from build123d import *

# Parameters (mm, degrees)
SALIENTE_EXTRUIR1_DEPTH = 1.25
SALIENTE_EXTRUIR2_DEPTH = 3.25
SALIENTE_EXTRUIR3_DEPTH = 5
SALIENTE_EXTRUIR4_DEPTH = 225.499987602
SALIENTE_EXTRUIR6_REACH = 368.413
CROQUIS6_W              = 4.5
CROQUIS6_H              = 225.499987602
CHAFL_N1_SIZE           = 0.6
CHAFL_N1_SIZE_2         = 0.279784595
REDONDEO1_R             = 0.5
CORTAR_EXTRUIR1_REACH   = 369.581
CROQUIS8_R              = 1.7
CORTAR_EXTRUIR2_DEPTH   = 409.723751009


with BuildPart() as part:
    # Croquis1 → Saliente-Extruir1 (new body)
    with BuildSketch(Plane.XY):
        Polygon((287.750005722, 59.751000255), (272.747904062, 59.751000255), (267.749905586, 64.749002457), (64.157357861, 64.749002457), (64.553998411, 290.248990059), (76.149903238, 290.248990059), (76.149903238, 77.348701656), (276.148021221, 77.348701656), (276.148021221, 290.248990059), (287.750005722, 290.248990059), align=None)
    extrude(amount=SALIENTE_EXTRUIR1_DEPTH)

    # Croquis2 → Saliente-Extruir2 (add)
    with BuildSketch(Plane.XY.offset(1.25)):
        Polygon((286.75003751, 290.248990059), (287.750005722, 290.248990059), (287.750005722, 59.751000255), (272.747904062, 59.751000255), (267.749905586, 64.749002457), (64.157357861, 64.749002457), (64.553998411, 290.248990059), (65.547994841, 290.248990059), (65.547994841, 66.199905073), (286.75003751, 66.199905073), align=None)
    extrude(amount=SALIENTE_EXTRUIR2_DEPTH)

    # Croquis3 → Saliente-Extruir3 (add)
    with BuildSketch(Plane.XZ.offset(-64.749002457)):
        with BuildLine():
            Line((64.515409591, 0), (66.982480076, 0))
            ThreePointArc((66.982480076, 0), (65.748944833, 2.619014625), (64.515409591, 0))
        make_face()
    extrude(amount=SALIENTE_EXTRUIR3_DEPTH)

    # Saliente-Extruir6: up to this face of the body (flat: up to its plane)
    saliente_extruir6_end = Plane(part.part.faces().sort_by_distance((64.355678136, 177.498996258, 2.25))[0])
    # Croquis6 → Saliente-Extruir6 (add, up to the picked face)
    with BuildSketch(Plane(origin=(64.157357861, 0, 0), x_dir=(0, 0, -1), z_dir=(1, 0, 0)), mode=Mode.PRIVATE) as saliente_extruir6_sk1:
        with Locations((-2.25, 177.498996258)):
            Rectangle(CROQUIS6_W, CROQUIS6_H)
    saliente_extruir6_tool1 = split(extrude(saliente_extruir6_sk1.sketch, amount=SALIENTE_EXTRUIR6_REACH, mode=Mode.PRIVATE), bisect_by=saliente_extruir6_end, keep=Keep.BOTH, mode=Mode.PRIVATE)


with BuildPart() as body_2:
    # Croquis3<3> → Saliente-Extruir4 (new body)
    with BuildSketch(Plane.XZ.offset(-64.749002457)):
        with BuildLine():
            Line((64.157357861, 3.992626763), (64.157357861, 0))
            ThreePointArc((64.157357861, 0), (62.24843494, 1.996313381), (64.157357861, 3.992626763))
        make_face()
    extrude(amount=-SALIENTE_EXTRUIR4_DEPTH)


with BuildPart() as part_1:
    add(part.part)

    add(body_2.part)  # Saliente-Extruir6 merges body 2
    add(saliente_extruir6_tool1.solids().sort_by(Axis((64.157358, 177.498996, 2.25), (1, 0, 0)))[0])

    # Chaflán1
    # the kernel refuses this chamfer: 0.6, 0.279784595 mm, written as the material it takes off along each edge
    with BuildSketch(Plane(origin=(64.157357861, 63.194417174, 4.5), x_dir=(-0.016311164131115618, 0, -0.9998669641130703), z_dir=(0, 1, 0))) as chafl_n1_piece_1_section:
        Polygon((CHAFL_N1_SIZE * 0.999866964113, -CHAFL_N1_SIZE * 0.0163111641311), (-CHAFL_N1_SIZE_2 * 0.0163111641249, -CHAFL_N1_SIZE_2 * 0.999866963731), (0, 0), align=None)
    chafl_n1_piece_1 = extrude(amount=228.609158168, mode=Mode.PRIVATE)
    chafl_n1_piece_1 = chafl_n1_piece_1 - Plane(origin=(64.246748688, 177.498996258, 1.996313381), x_dir=(-0.044733129364357686, 0, -0.9989989725406486), z_dir=(0, -1, 0)) * Cylinder(1.998313748, 460, mode=Mode.PRIVATE)
    add(chafl_n1_piece_1, mode=Mode.SUBTRACT)

    # Redondeo1
    redondeo1_edges = [part_1.edges().sort_by_distance(p)[0] for p in [
        (65.748944833, 64.749002457, 2.619014625),
    ]]
    fillet(redondeo1_edges, radius=REDONDEO1_R)

    # Cortar-Extruir1: up to this plane
    cortar_extruir1_end = Plane(origin=(272.747904062, 59.751000255, 1.25), z_dir=(0.7071070447096931, 0.7071065176633039, 0))
    # Croquis7 → Cortar-Extruir1 (cut, up to the surface)
    with BuildSketch(Plane(origin=(287.750005722, 0, 0), x_dir=(0, 0, -1), z_dir=(1, 0, 0)), mode=Mode.PRIVATE) as cortar_extruir1_sk1:
        Polygon((-2, 59.751000255), (-4.5, 64.749002457), (-4.5, 59.751000255), align=None)
    cortar_extruir1_tool1 = split(extrude(cortar_extruir1_sk1.sketch, amount=-CORTAR_EXTRUIR1_REACH, mode=Mode.PRIVATE), bisect_by=cortar_extruir1_end, keep=Keep.BOTH, mode=Mode.PRIVATE)
    add(cortar_extruir1_tool1.solids().sort_by_distance((287.750006, 61.417001, 3.666667))[0], mode=Mode.SUBTRACT)

    # Croquis8 → Cortar-Extruir2 (cut, through all)
    with BuildSketch(Plane.XY.offset(1.25)):
        with Locations((176.148989202, 71.774303364)):
            Circle(CROQUIS8_R)
        with Locations((91.149903238, 71.774303364)):
            Circle(CROQUIS8_R)
        with Locations(Location((261.148075163, 71.775125937, 0), (0, 0, 180))):
            Circle(CROQUIS8_R)
        with Locations((70.848949039, 92.348701656)):
            Circle(CROQUIS8_R)
        with Locations((70.848949039, 122.348701656)):
            Circle(CROQUIS8_R)
        with Locations((70.848949039, 275.248990059)):
            Circle(CROQUIS8_R)
        with Locations((70.848949039, 198.798845857)):
            Circle(CROQUIS8_R)
        with Locations(Location((281.44853993, 122.349720687, 0), (0, 0, 180))):
            Circle(CROQUIS8_R)
        with Locations(Location((281.447800089, 198.799864885, 0), (0, 0, 180))):
            Circle(CROQUIS8_R)
        with Locations(Location((281.447060248, 275.250009083, 0), (0, 0, 180))):
            Circle(CROQUIS8_R)
        with Locations(Location((281.448830253, 92.349720689, 0), (0, 0, 180))):
            Circle(CROQUIS8_R)
    extrude(amount=-CORTAR_EXTRUIR2_DEPTH, mode=Mode.SUBTRACT)


solid = part_1.part
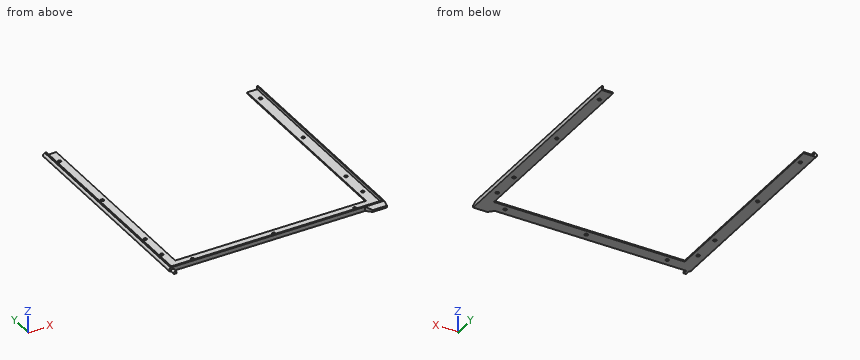
Can you work these out from the model? Positions are in its coordinate system, mm. Coordinates: 2 decimals unless noted, no trailing zeros. Write each loop counter-clockwise with the first axis right and the second up, starting at its lowest first coordinate (ties: lowest second). Pieces come first, ordered by that corner, then holes. Notation, with made-up numbers: (21.5, 38.25) - (58.5, 38.25) arc R27 cw to (58.5, 57.25) - close; hole circle Ø4 at (62.25, -23). An arc over 180 degrees is marked (long way). Return JSON: item names as keys, results as strings. Group by question number.
Item 1: Please list where these lines run through material, in increasing order: probe 1 along Y at (x, z) = (109.5, 2.6); probe 2 along Z at (x, y) = (112.5, 77); probe 3 along X at (y, z) = (160.5, 1.7).
Item 2: If we section it at A-A (y = 144): Write out the boundary of the cut face in (x, z).
Item 3: If we section it at B-B (x = 137.5): Write out the boundary of the cut face in (y, z).
Item 4: I'm going to push flat-ended pins straight in: pin 1 Ø3 at (x, y) = (70.85, 198.8) entering from -Z; pin 2 Ø2 at (x, z) = (176, 3) entering from -Y; pin 3 Ø4 at (x, y) = (281.45, 198.8) entering from +Z; pin 4 Ø2.5 at (x, z) = (180.5, 3.5) entering from +Y. Where does each tip first touch, or does it pass through?
Return value:
{
 "1": {"probe 1": "y = 64.75 to 66.2", "probe 2": "z = 0 to 1.25", "probe 3": "x = 62.27 to 65.55, 286.75 to 287.75"},
 "2": {"outline": "(64.16, 0) - (76.15, 0) - (76.15, 1.25) - (65.55, 1.25) - (65.55, 4.5) - (64.44, 4.5) - (64.2, 3.99) arc R2 ccw to start; (276.15, 0) - (287.75, 0) - (287.75, 4.5) - (286.75, 4.5) - (286.75, 1.25) - (276.15, 1.25) - close"},
 "3": {"outline": "(64.75, 0) - (77.35, 0) - (77.35, 1.25) - (66.2, 1.25) - (66.2, 4.5) - (64.75, 4.5) - close"},
 "4": {"pin 1": "passes through", "pin 2": "stops at y = 64.75", "pin 3": "stops at z = 1.25", "pin 4": "stops at y = 66.2"}
}
